```python
from build123d import *

# Parameters (mm, degrees)
SKETCH_11_W         = 15
SKETCH_11_H         = 15
SKETCH_11_W_2       = 13
SKETCH_11_H_2       = 13
F_15X15X1_1_DEPTH   = 170
SKETCH_13_R         = 1.45
CUT_EXTRUDE_2_DEPTH = 87.638617256
SKETCH_14_R         = 1.45
CUT_EXTRUDE_3_DEPTH = 87.638617256


with BuildPart() as part:
    # 草图11 → 铝管 15X15X1(1) (new body)
    with BuildSketch(Plane(origin=(-85, 0, 0), x_dir=(0, 0, -1), z_dir=(1, 0, 0))):
        Rectangle(SKETCH_11_W, SKETCH_11_H)
        Rectangle(SKETCH_11_W_2, SKETCH_11_H_2, mode=Mode.SUBTRACT)
    extrude(amount=F_15X15X1_1_DEPTH)

    # 草图13 → 切除-拉伸2 (cut, through all)
    with BuildSketch(Plane(origin=(0, 7.5, 0), x_dir=(1, 0, 0), z_dir=(0, 1, 0))):
        with Locations(Location((-80, 0, 0), (0, 0, 270))):
            Circle(SKETCH_13_R)
        with Locations(Location((-70, 0, 0), (0, 0, 270))):
            Circle(SKETCH_13_R)
        with Locations(Location((70, 0, 0), (0, 0, 90))):
            Circle(SKETCH_13_R)
        with Locations(Location((80, 0, 0), (0, 0, 90))):
            Circle(SKETCH_13_R)
    extrude(amount=-CUT_EXTRUDE_2_DEPTH, mode=Mode.SUBTRACT)

    # 草图14 → 切除-拉伸3 (cut, through all)
    with BuildSketch(Plane(origin=(0, 7.5, 0), x_dir=(1, 0, 0), z_dir=(0, 1, 0))):
        with Locations(Location((-20, 0, 0), (0, 0, 270))):
            Circle(SKETCH_14_R)
        with Locations(Location((20, 0, 0), (0, 0, 270))):
            Circle(SKETCH_14_R)
    extrude(amount=-CUT_EXTRUDE_3_DEPTH, mode=Mode.SUBTRACT)


solid = part.part
```
Source: CAD feature listing. Evaluate the final solid. Frame: model axes, mm. A direction names the side the tool comes from. Round coordinates to 2 decimals unless told otherwise and drop trailing zeros. Write each loop counter-clockwise with the first axis right and the second up, starting at its lowest first coordinate (ties: lowest second). Pieces come first, ordered by that corner, then holes. Notation, with made-up numbers: M 9,3.25 L 21,3.25 A26 cw 21,19.25 Z; hole C 64.5,2.5 d7. An arc over 180 degrees is marked long. Use CSV: the item, a comma, the result in double quotes. Start each with the question number.
Q1. Cut plane D-D on x = 12. Output: boundary loops of the cut face in (y, z).
Q2. Access query for faces 1 (the face through (-1, 7.5, 0)), 2 (the face through (-1, 0, -6.5)). Directions: +Z, -Z, +X, -X, +Y, -Y. A direction counts if a zero-diameter tool reaches every point of the face in a straight line with its end or side. Return the directions, or none.
Q3. Pull-direction query (X, two-part tool) for faces 3 (the face through (-1, 6.5, 0)), 4 (the face through (85, 0, 7)), 5 (the face through (81.416, 7.007, 0.314)); classes: +X half, -X half, draft (parallel to the pull), parting line (faces both ways), or undercut.
Q4. Line query: line 1 (Z direction, x = 10.5, y = -4); line 2 (Z direction, x = 80, y = -7.2). Output: solid intervals per line, ascending. Write a range as from..to.
Q5. Cut plane C-C on x = -70. Output: boundary loops of the cut face in (y, z), plus the area to 3 significant figures.
Q6. Cut plane A-A on z = -4.25. Output: boundary loops of the cut face in (x, y).
Results found:
1,outline,"M -7.5,-7.5 L 7.5,-7.5 L 7.5,7.5 L -7.5,7.5 Z; hole M -6.5,-6.5 L 6.5,-6.5 L 6.5,6.5 L -6.5,6.5 Z"
2,face 1,"+Z, -Z, +X, -X, +Y"
2,face 2,"+X, -X"
3,face 3,"draft"
3,face 4,"+X half"
3,face 5,"undercut"
4,line 1,"-7.5..-6.5, 6.5..7.5"
4,line 2,"-7.5..-1.45, 1.45..7.5"
5,outline,"M -7.5,-7.5 L 7.5,-7.5 L 7.5,-1.45 L 6.5,-1.45 L 6.5,-6.5 L -6.5,-6.5 L -6.5,-1.45 L -7.5,-1.45 Z; M -7.5,1.45 L -6.5,1.45 L -6.5,6.5 L 6.5,6.5 L 6.5,1.45 L 7.5,1.45 L 7.5,7.5 L -7.5,7.5 Z"
5,area,"50.2 mm^2"
6,outline,"M -85,-7.5 L 85,-7.5 L 85,-6.5 L -85,-6.5 Z; M -85,6.5 L 85,6.5 L 85,7.5 L -85,7.5 Z"
